Part model, mm, in its own coordinate system. Face numbers are marked on the shaded views. A direction names the side the tool comes from. Round coordinates to 2 decimals unless told otherwise and drop trailing zeros. Write each loop counter-clockwise with the first axis right and the second up, starting at its lowest first coordinate (ties: lowest second). Pieces come first, ordered by that corner, then holes.
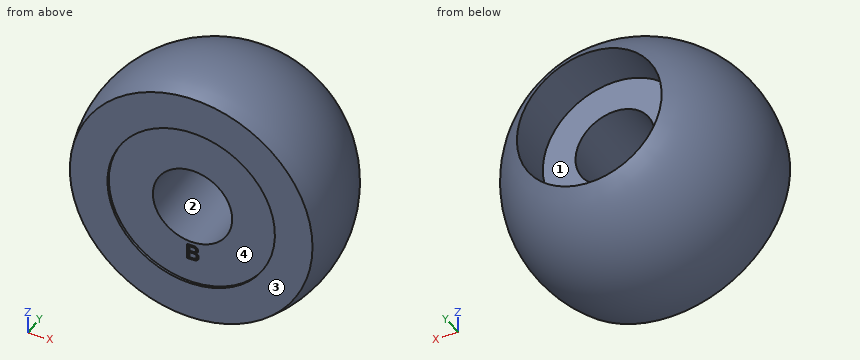
```python
from build123d import *

# Parameters (mm, degrees)
TRUNCATED_BALL_DEPTH      = 11.998522628
TRUNCATED_BALL_DEPTH_BACK = 11.998522628
SKETCH3_R                 = 4.1275
RECESSED_DEPTH            = 0.127
CUT_EXTRUDE1_DEPTH        = 0.127


with BuildPart() as part:
    # Sketch1 → Complete_Ball (revolve)
    with BuildSketch(Plane.XY):
        with BuildLine():
            Line((0, 6.35), (0, -6.35))
            ThreePointArc((0, -6.35), (6.35, 0), (0, 6.35))
        make_face()
    revolve(axis=Axis((0, 5.621617492, 0), (0, -1, 0)))

    # Sketch2 → Truncated_ball (cut, two sides)
    with BuildSketch(Plane.XY) as truncated_ball_sk:
        with BuildLine():
            Line((-5.980823609, -2.1336), (5.980823609, -2.1336))
            ThreePointArc((5.980823609, -2.1336), (0, -6.35), (-5.980823609, -2.1336))
        make_face()
    extrude(amount=TRUNCATED_BALL_DEPTH, mode=Mode.SUBTRACT)
    extrude(truncated_ball_sk.sketch, amount=-TRUNCATED_BALL_DEPTH_BACK, mode=Mode.SUBTRACT)

    # Sketch3 → Recessed (cut)
    with BuildSketch(Plane.XZ.offset(2.1336)):
        with Locations(Location((0, 0, 0), (0, 0, 270))):
            Circle(SKETCH3_R)
    extrude(amount=-RECESSED_DEPTH, mode=Mode.SUBTRACT)

    # Sketch5 → Counterbored_hole (revolve, cut)
    with BuildSketch(Plane.XY, mode=Mode.PRIVATE) as counterbored_hole_sk:
        Polygon((1.9558, -2.1336), (1.9558, 2.8448), (3.5687, 2.8448), (3.5687, 6.35), (0, 6.35), (0, -2.1336), align=None)
    revolve(counterbored_hole_sk.sketch.rotate(Axis((0, 7.818373071, 0), (0, -1, 0)), 90), axis=Axis((0, 7.818373071, 0), (0, -1, 0)), mode=Mode.SUBTRACT)

    # Sketch9 → Cut-Extrude1 (cut)
    with BuildSketch(Plane.XZ.offset(2.0066)):
        with BuildLine():
            Line((-0.266710017, -2.9083), (-0.266710017, -2.137804395))
            Line((-0.266710017, -2.137804395), (0.021762797, -2.137804395))
            add(Edge.make_bspline(
                [(0.021762797, -2.137804395), (0.028916445, -2.137831838), (0.042875247, -2.137885387), (0.063257985, -2.1392246), (0.08256196, -2.141056366), (0.100828728, -2.143417569), (0.117979251, -2.146843626), (0.133997544, -2.150994066), (0.148966969, -2.155781463), (0.167264808, -2.16307422), (0.188351063, -2.174299324), (0.210936444, -2.19104895), (0.230586604, -2.211159242), (0.246755795, -2.234216831), (0.260077465, -2.258846684), (0.269522373, -2.28457958), (0.275561015, -2.31085525), (0.276246169, -2.328647268), (0.276588166, -2.337528215)],
                knots=[0, 0, 0, 0, 0.939712594, 1.833646414, 2.682508961, 3.487467313, 4.25240329, 4.978730417, 5.660668875, 6.315918528, 7.564895217, 8.787077865, 9.996481721, 11.241996224, 12.475862915, 13.665015424, 14.834484263, 16, 16, 16, 16], degree=3))
            add(Edge.make_bspline(
                [(0.276588166, -2.337528215), (0.276228655, -2.345790733), (0.275513098, -2.362236109), (0.269818069, -2.386461149), (0.260829571, -2.409983511), (0.24811958, -2.432517235), (0.231874618, -2.453650072), (0.211735504, -2.472667007), (0.187991636, -2.489608795), (0.170171864, -2.498639265), (0.160982956, -2.5032959)],
                knots=[0, 0, 0, 0, 0.926741525, 1.844548388, 2.778836836, 3.746021974, 4.738420572, 5.759761325, 6.844803049, 8, 8, 8, 8], degree=3))
            add(Edge.make_bspline(
                [(0.160982956, -2.5032959), (0.166667275, -2.505075335), (0.177796205, -2.508559168), (0.193795198, -2.514934092), (0.208813366, -2.522192856), (0.2228834, -2.530347388), (0.23591023, -2.539473202), (0.2478571, -2.549584525), (0.258806843, -2.560524888), (0.268739897, -2.572287634), (0.277465043, -2.58479707), (0.285290409, -2.597779786), (0.291752256, -2.611392125), (0.297048797, -2.625598745), (0.301180886, -2.640311862), (0.304148175, -2.655588064), (0.305839455, -2.671391794), (0.306093479, -2.68212759), (0.306222612, -2.687585113)],
                knots=[0, 0, 0, 0, 1.127427615, 2.20731145, 3.257257018, 4.283066884, 5.282973838, 6.264540225, 7.242620376, 8.210460609, 9.17525685, 10.12748095, 11.077310519, 12.023587065, 12.994999128, 13.967387486, 14.966724908, 16, 16, 16, 16], degree=3))
            add(Edge.make_bspline(
                [(0.306222612, -2.687585113), (0.30595645, -2.69634709), (0.305428882, -2.713714396), (0.301191929, -2.739276148), (0.294031702, -2.7638644), (0.28417626, -2.787081588), (0.272433103, -2.808549297), (0.259086593, -2.827705432), (0.244477096, -2.844352877), (0.22819322, -2.858356354), (0.210340006, -2.870241208), (0.190413202, -2.880249032), (0.168566879, -2.889074974), (0.144357023, -2.896125462), (0.117794653, -2.901726361), (0.088519295, -2.905365274), (0.056485971, -2.907970248), (0.034167963, -2.908187011), (0.022534527, -2.9083)],
                knots=[0, 0, 0, 0, 1.028073207, 2.037766189, 3.031549473, 4.027532207, 4.992436545, 5.898794514, 6.762903869, 7.584966804, 8.412380356, 9.273953678, 10.198004568, 11.174406109, 12.229717296, 13.381036288, 14.634844708, 16, 16, 16, 16], degree=3))
            Line((0.022534527, -2.9083), (-0.266710017, -2.9083))
        make_face()
        with BuildLine():
            Line((-0.158050381, -2.463783305), (0.00077173, -2.463783305))
            add(Edge.make_bspline(
                [(0.00077173, -2.463783305), (0.005968785, -2.463762743), (0.015953502, -2.46372324), (0.030356217, -2.463172446), (0.043649233, -2.46270254), (0.055781131, -2.461523111), (0.066812012, -2.460367914), (0.076697733, -2.458812838), (0.085486714, -2.45706062), (0.090868209, -2.455435306), (0.093379375, -2.454676886)],
                knots=[0, 0, 0, 0, 1.335841395, 2.566453063, 3.705076039, 4.753984432, 5.69893722, 6.555639608, 7.326018133, 8, 8, 8, 8], degree=3))
            add(Edge.make_bspline(
                [(0.093379375, -2.454676886), (0.099279717, -2.452609996), (0.11065434, -2.448625465), (0.125897399, -2.439576193), (0.138880055, -2.428717112), (0.149567516, -2.415856475), (0.157780301, -2.401063109), (0.163869844, -2.384643791), (0.167204004, -2.366368995), (0.167680456, -2.353696066), (0.167928529, -2.347097672)],
                knots=[0, 0, 0, 0, 1.059015028, 2.041559358, 2.989777133, 3.920090524, 4.862499371, 5.848878527, 6.879979022, 8, 8, 8, 8], degree=3))
            add(Edge.make_bspline(
                [(0.167928529, -2.347097672), (0.167729061, -2.340756189), (0.167340322, -2.328397369), (0.164077197, -2.31045022), (0.158430481, -2.293753694), (0.150783282, -2.278311452), (0.141099895, -2.264573361), (0.129542435, -2.252761818), (0.115697414, -2.243832811), (0.102756467, -2.238262878), (0.09111711, -2.23477836), (0.080717754, -2.232716714), (0.068921782, -2.230900199), (0.055690377, -2.229355858), (0.041018534, -2.228157307), (0.024861047, -2.227205138), (0.007256378, -2.22680087), (-0.00493898, -2.226739552), (-0.011267263, -2.226707734)],
                knots=[0, 0, 0, 0, 1.216168307, 2.37017178, 3.484610845, 4.588286376, 5.664695412, 6.69777344, 7.738183022, 8.803673002, 9.390844981, 10.0665252, 10.835811589, 11.680682236, 12.621801058, 13.660007223, 14.785756265, 16, 16, 16, 16], degree=3))
            Line((-0.011267263, -2.226707734), (-0.158050381, -2.226707734))
            Line((-0.158050381, -2.226707734), (-0.158050381, -2.463783305))
        make_face(mode=Mode.SUBTRACT)
        with BuildLine():
            Line((-0.158050381, -2.819396661), (0.024232334, -2.819396661))
            add(Edge.make_bspline(
                [(0.024232334, -2.819396661), (0.031486765, -2.819313318), (0.044815157, -2.819160193), (0.063045794, -2.818679835), (0.077781785, -2.817506499), (0.086386824, -2.816243115), (0.090138108, -2.815692355)],
                knots=[0, 0, 0, 0, 1.317581857, 2.420761387, 3.311546315, 4, 4, 4, 4], degree=3))
            add(Edge.make_bspline(
                [(0.090138108, -2.815692355), (0.095516334, -2.814561906), (0.105929971, -2.812373065), (0.120610701, -2.807487801), (0.134071074, -2.80189147), (0.14607616, -2.794779154), (0.157192582, -2.786582698), (0.16685358, -2.776344933), (0.175751817, -2.764713097), (0.183461357, -2.751401785), (0.189695639, -2.736675926), (0.194460394, -2.720763047), (0.19699845, -2.703718942), (0.197372145, -2.692017237), (0.197562976, -2.686041652)],
                knots=[0, 0, 0, 0, 1.067651492, 2.067249321, 3.003744366, 3.895862395, 4.774133402, 5.679610569, 6.621910665, 7.616993802, 8.661192143, 9.724711987, 10.838102842, 12, 12, 12, 12], degree=3))
            add(Edge.make_bspline(
                [(0.197562976, -2.686041652), (0.197350369, -2.679025957), (0.196935765, -2.665344636), (0.192994812, -2.645574434), (0.186485001, -2.627237325), (0.177321084, -2.610587261), (0.166081062, -2.595611962), (0.15248177, -2.582908823), (0.136624895, -2.572828254), (0.118461703, -2.564916959), (0.09723257, -2.559288208), (0.072351402, -2.555469442), (0.043420216, -2.553005284), (0.02274604, -2.552797406), (0.011730302, -2.552686644)],
                knots=[0, 0, 0, 0, 0.96167883, 1.875371887, 2.752872588, 3.621584364, 4.472914353, 5.312011319, 6.159851575, 7.038572308, 8.019870099, 9.164119506, 10.488969081, 12, 12, 12, 12], degree=3))
            Line((0.011730302, -2.552686644), (-0.158050381, -2.552686644))
            Line((-0.158050381, -2.552686644), (-0.158050381, -2.819396661))
        make_face(mode=Mode.SUBTRACT)
    extrude(amount=-CUT_EXTRUDE1_DEPTH, mode=Mode.SUBTRACT)


solid = part.part
```
Q1. Cut at C-C on x = 5. Write the cut outline in (y, z).
Values follow:
outline: (-2.13, -3.28) arc R3.91 ccw (long way) to (-2.13, 3.28) - close
Q2. Wall check: L1, parallel to X at y = 4.35, z = 0; L2, parallel to X at y = 1.75, z = 1.75; L3, parallel to Y at x = 1.5, z = -2.75. Give the ranges that are in metal, low to high.
Values follow:
L1: x = -4.63 to -3.57, 3.57 to 4.63
L2: x = -5.85 to -0.87, 0.87 to 5.85
L3: y = -2.01 to 2.84
Q3. Mould opens along X. For the marked faces 3 and 4 say: +X half, -X half, draft (parallel to the pull), parting line (faces both ways), or undercut.
Values follow:
face 3: draft
face 4: undercut
Q4. Which spindle directions (+Z, -Z, +X, -X, +Y, -Y) get a long thin tool onto all of the face, cutting with end or side? Do the marked faces 1 and 2. Say none if no direction does.
Values follow:
face 1: +Y
face 2: +Y, -Y
Q5. Drop flat-ended pins along their axis: pin 1 (4 mm diameter, centred on x = -0.5, z = -0.5, fed in from -Y); pin 2 (4 mm diameter, centred on x = 1, y = 3, fed in from +Z); pin 3 (2 mm diameter, centred on x = -0.5, z = 0, fed in from +Y); pin 4 (1.5 mm diameter, centred on y = -0.5, z = -1, fed in from +X). Give the stop position or say it passes through.
Values follow:
pin 1: stops at y = -2.01
pin 2: stops at z = 6.24
pin 3: passes through
pin 4: stops at x = 6.34
Q6. Cut at D-D on z = 5.25. Write the cut outline in (x, y), plus the area to 3 significant figures.
Values follow:
outline: (-2.86, -2.13) - (2.86, -2.13) arc R3.57 ccw (long way) to start
area: 34.3 mm2
Q7. Cut at A-A on z = 0. Write the cut outline in (x, y).
Values follow:
outline: (-5.98, -2.13) - (-4.13, -2.13) - (-4.13, -2.01) - (-1.96, -2.01) - (-1.96, 2.84) - (-3.57, 2.84) - (-3.57, 5.25) arc R6.35 ccw to start; (1.96, -2.01) - (4.13, -2.01) - (4.13, -2.13) - (5.98, -2.13) arc R6.35 ccw to (3.57, 5.25) - (3.57, 2.84) - (1.96, 2.84) - close
Q8. Cut at B-B on y = 0. Write the cut outline in (x, z).
Values follow:
outline: circle Ø12.7 at (0, 0); hole circle Ø3.91 at (0, 0)
